Geometry: final body of the model. Coordinates: model frame, mm. Face numbers are marked on the shaded views. A direction names the side the tool comes from. Give positions to 0.01 mm unless a question says otherwise; leave off trailing zeros. Write each loop counter-clockwise with the first axis right and the second up, starting at its lowest first coordinate (ties: lowest second). Pieces come first, ordered by that corner, then holes.
from build123d import *

# Parameters (mm, degrees)
SKETCH10_R          = 37
BOSS_EXTRUDE1_DEPTH = 50
SKETCH11_R          = 2.5
CUT_EXTRUDE1_DEPTH  = 25


with BuildPart() as part:
    # Sketch3 → Revolve1 (revolve)
    with BuildSketch(Plane.XY):
        with BuildLine():
            Line((0, 0), (200, 0))
            Line((200, 0), (200, 38.1))
            add(Edge.make_bspline(
                [(0, 0), (0.333278549, 0.131540873), (0.999577039, 0.394520549), (1.999623692, 0.786334891), (2.999614377, 1.17601578), (4.66502861, 1.821148753), (7.328741847, 2.840985756), (11.325969227, 4.339896645), (15.327567951, 5.800346847), (21.648365914, 8.05135545), (32.594864134, 11.782666432), (44.617809557, 15.495925888), (54.658642309, 18.334838057), (59.993667814, 19.782959156), (64.329338058, 20.915666696), (68.662820277, 22.01269926), (73.990330688, 23.318521745), (78.993971117, 24.479998264), (83.997331558, 25.591796678), (87.330083915, 26.309365893), (93.324657038, 27.552988579), (99.987226118, 28.850738677), (109.652181507, 30.574297106), (118.320286798, 31.962202042), (124.997544263, 32.910660178), (132.98954992, 33.985397902), (141.318339795, 34.97224064), (150.663527404, 35.869691178), (156.997734153, 36.407242182), (166.989872456, 37.153259543), (176.661040051, 37.642869627), (186.332724985, 37.936353666), (190.666251166, 38.027993755), (194.333291829, 38.071814955), (195.999993248, 38.085597183), (196.999994924, 38.092040964), (197.999996625, 38.09660679), (198.999998309, 38.099469797), (199.666666479, 38.099823266), (200, 38.1)],
                knots=[0, 0, 0, 0, 0.005248402, 0.010492732, 0.015733018, 0.020969291, 0.036654322, 0.057513275, 0.083502072, 0.099051411, 0.155796901, 0.252897726, 0.283342643, 0.308639705, 0.333872761, 0.348983013, 0.37411934, 0.414220017, 0.424223641, 0.44919678, 0.464156839, 0.513902353, 0.54862082, 0.607960951, 0.642483277, 0.647409944, 0.726082727, 0.765324507, 0.784925615, 0.819199979, 0.912095095, 0.926749999, 0.960936877, 0.975586084, 0.980468966, 0.985351783, 0.990234549, 0.995117283, 1, 1, 1, 1], degree=3))
        make_face()
    revolve(axis=Axis((0, 0, 0), (1, 0, 0)))

    # Sketch10 → Boss-Extrude1 (add)
    with BuildSketch(Plane(origin=(200, 0, 0), x_dir=(0, 0, -1), z_dir=(1, 0, 0))):
        with Locations(Location((0, 0, 0), (0, 0, 180))):
            Circle(SKETCH10_R)
    extrude(amount=BOSS_EXTRUDE1_DEPTH)

    # Sketch11 → Cut-Extrude1 (cut)
    with BuildSketch(Plane(origin=(250, 0, 0), x_dir=(0, 0, -1), z_dir=(1, 0, 0))):
        Circle(SKETCH11_R)
    extrude(amount=-CUT_EXTRUDE1_DEPTH, mode=Mode.SUBTRACT)


solid = part.part
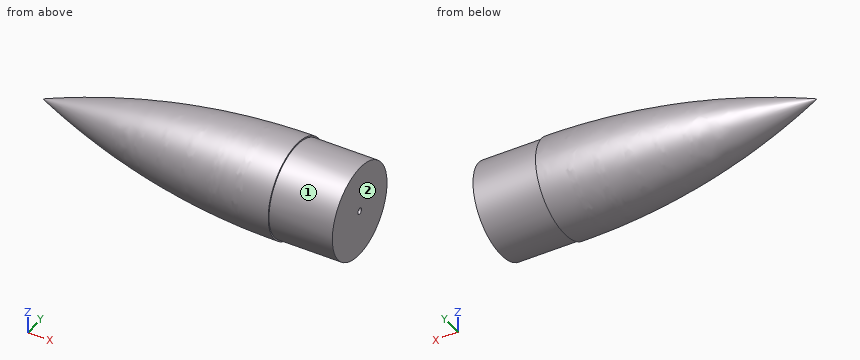
Q1. Access query for the marked faces 1 and 2. Directions: +Z, -Z, +X, -X, +Y, -Y. A direction counts if a zero-diameter tool reaches every point of the face in a straight line with its end or side. Return the directions, or none.
Filled sheet:
face 1: +X
face 2: +Z, -Z, +X, +Y, -Y
Q2. Ray query, line 1 along Y through (x, z) = (243.5, 0); line 2 along Z through (x, y) = (217, -1); line 3 along Z through (x, y) = (118.5, 12.5). Return the intervals inside material, ascending.
Filled sheet:
line 1: y = -37 to -2.5, 2.5 to 37
line 2: z = -36.99 to 36.99
line 3: z = -29.41 to 29.41
Q3. Section A-A on x = 215.5. Output: boundary loops of the cut face in (y, z).
Filled sheet:
outline: circle Ø74 at (0, 0)
Q4. Pin query (flat end, axial travel): P1, Ø4, axis at x = 203, y = -28.5, coming from the -Z side; P2, Ø1.5, axis at y = 1, z = -1, coming from the +X side; P3, Ø1, axis at x = 202.5, z = -1, coming from the -Y side; P4, Ø8, axis at y = 0, z = 0, coming from the -X side. Return the tip coordinate at first contact, or that it passes through.
Filled sheet:
P1: stops at z = -25.82
P2: stops at x = 225
P3: stops at y = -37
P4: stops at x = 0
